```python
from build123d import *

# Parameters (mm, degrees)
BOSS_EXTRUDE1_DEPTH = 12.4
SKETCH2_R           = 1.5
CUT_EXTRUDE1_DEPTH  = 46.584756224
CUT_EXTRUDE2_DEPTH  = 2
CUT_EXTRUDE3_START  = -2
CUT_EXTRUDE3_DEPTH  = 2
CUT_EXTRUDE4_DEPTH  = 1
CUT_EXTRUDE5_START  = -1
CUT_EXTRUDE5_DEPTH  = 1
CUT_EXTRUDE6_DEPTH  = 0.5
SKETCH9_R           = 4.5
BOSS_EXTRUDE2_DEPTH = 0.5
SKETCH10_R          = 4.25
BOSS_EXTRUDE3_DEPTH = 0.5
SKETCH11_R          = 4.5
BOSS_EXTRUDE4_DEPTH = 1
SKETCH12_R          = 3
BOSS_EXTRUDE5_DEPTH = 1
SKETCH13_R          = 2
BOSS_EXTRUDE6_DEPTH = 3
BOSS_EXTRUDE7_DEPTH = 5


with BuildPart() as part:
    # Sketch1 → Boss-Extrude1 (new body)
    with BuildSketch(Plane(origin=(0, 0, 0), x_dir=(0, 0, -1), z_dir=(1, 0, 0))):
        with BuildLine():
            Line((1, 0), (27.9, 0))
            ThreePointArc((27.9, 0), (28.607106781, -0.292893219), (28.9, -1))
            Line((28.9, -1), (28.9, -24.904637595))
            ThreePointArc((28.9, -24.904637595), (28.813500063, -25.31147618), (28.568964732, -25.647931742))
            Line((28.568964732, -25.647931742), (20.685228726, -32.743294146))
            ThreePointArc((20.685228726, -32.743294146), (20.374527762, -32.933620412), (20.016263995, -33))
            Line((20.016263995, -33), (1, -33))
            ThreePointArc((1, -33), (0.292893219, -32.707106781), (0, -32))
            Line((0, -32), (0, -1))
            ThreePointArc((0, -1), (0.292893219, -0.292893219), (1, 0))
        make_face()
    extrude(amount=BOSS_EXTRUDE1_DEPTH)

    # Sketch2 → Cut-Extrude1 (cut, through all)
    with BuildSketch(Plane(origin=(12.4, 0, 0), x_dir=(0, 0, -1), z_dir=(1, 0, 0))):
        with Locations((25.9, -3)):
            Circle(SKETCH2_R)
        with Locations((9.9, -30)):
            Circle(SKETCH2_R)
    extrude(amount=-CUT_EXTRUDE1_DEPTH, mode=Mode.SUBTRACT)

    # Sketch3 → Cut-Extrude2 (cut)
    with BuildSketch(Plane(origin=(12.4, 0, 0), x_dir=(0, 0, -1), z_dir=(1, 0, 0))):
        with BuildLine():
            Line((6.9, -30), (6.9, -32.602246067))
            Line((6.9, -32.602246067), (0, -32.602246067))
            Line((0, -32.602246067), (0, -33))
            Line((0, -33), (6.9, -33))
            Line((6.9, -33), (12.9, -33))
            Line((12.9, -33), (12.9, -30))
            ThreePointArc((12.9, -30), (9.9, -27), (6.9, -30))
        make_face()
        with BuildLine():
            Line((22.9, 0), (28.9, 0))
            Line((28.9, 0), (28.9, -6))
            Line((28.9, -6), (25.9, -6))
            ThreePointArc((25.9, -6), (23.778679656, -5.121320344), (22.9, -3))
            Line((22.9, -3), (22.9, 0))
        make_face()
    extrude(amount=-CUT_EXTRUDE2_DEPTH, mode=Mode.SUBTRACT)

    # Sketch4 → Cut-Extrude3 (cut)
    with BuildSketch(Plane.ZY.offset(CUT_EXTRUDE3_START)):
        with BuildLine():
            Line((-12.9, -30), (-12.9, -33))
            Line((-12.9, -33), (-6.9, -33))
            Line((-6.9, -33), (0, -33))
            Line((0, -33), (0, -32.6))
            Line((0, -32.6), (-6.9, -32.6))
            Line((-6.9, -32.6), (-6.9, -30))
            ThreePointArc((-6.9, -30), (-9.9, -27), (-12.9, -30))
        make_face()
        with BuildLine():
            Line((-28.9, 0), (-22.9, 0))
            Line((-22.9, 0), (-22.9, -3))
            ThreePointArc((-22.9, -3), (-23.778679656, -5.121320344), (-25.9, -6))
            Line((-25.9, -6), (-28.9, -6))
            Line((-28.9, -6), (-28.9, 0))
        make_face()
    extrude(amount=CUT_EXTRUDE3_DEPTH, mode=Mode.SUBTRACT)

    # Sketch5 → Cut-Extrude4 (cut)
    with BuildSketch(Plane(origin=(12.4, 0, 0), x_dir=(0, 0, -1), z_dir=(1, 0, 0))):
        with BuildLine():
            Line((5, -3), (5, -25))
            ThreePointArc((5, -25), (5.292893219, -25.707106781), (6, -26))
            Line((6, -26), (10.9, -26))
            ThreePointArc((10.9, -26), (13.021320344, -26.878679656), (13.9, -29))
            Line((13.9, -29), (13.9, -30))
            Line((13.9, -30), (15.875361746, -30))
            ThreePointArc((15.875361746, -30), (16.233625514, -29.933620412), (16.544326478, -29.743294146))
            Line((16.544326478, -29.743294146), (27.068964732, -20.271119718))
            ThreePointArc((27.068964732, -20.271119718), (27.313500063, -19.934664157), (27.4, -19.527825572))
            Line((27.4, -19.527825572), (27.4, -8))
            ThreePointArc((27.4, -8), (27.107106781, -7.292893219), (26.4, -7))
            Line((26.4, -7), (24.9, -7))
            ThreePointArc((24.9, -7), (22.778679656, -6.121320344), (21.9, -4))
            Line((21.9, -4), (21.9, -3))
            ThreePointArc((21.9, -3), (21.607106781, -2.292893219), (20.9, -2))
            Line((20.9, -2), (6, -2))
            ThreePointArc((6, -2), (5.292893219, -2.292893219), (5, -3))
        make_face()
    extrude(amount=-CUT_EXTRUDE4_DEPTH, mode=Mode.SUBTRACT)

    # Sketch6 → Cut-Extrude5 (cut)
    with BuildSketch(Plane.ZY.offset(CUT_EXTRUDE5_START)):
        with BuildLine():
            Line((-6, -2), (-20.9, -2))
            ThreePointArc((-20.9, -2), (-21.607106781, -2.292893219), (-21.9, -3))
            Line((-21.9, -3), (-21.9, -4))
            ThreePointArc((-21.9, -4), (-22.778679656, -6.121320344), (-24.9, -7))
            Line((-24.9, -7), (-26.4, -7))
            ThreePointArc((-26.4, -7), (-27.107106781, -7.292893219), (-27.4, -8))
            Line((-27.4, -8), (-27.4, -19.527825572))
            ThreePointArc((-27.4, -19.527825572), (-27.313500063, -19.934664157), (-27.068964732, -20.271119718))
            Line((-27.068964732, -20.271119718), (-16.544326478, -29.743294146))
            ThreePointArc((-16.544326478, -29.743294146), (-16.233625514, -29.933620412), (-15.875361746, -30))
            Line((-15.875361746, -30), (-13.9, -30))
            Line((-13.9, -30), (-13.9, -29))
            ThreePointArc((-13.9, -29), (-13.021320344, -26.878679656), (-10.9, -26))
            Line((-10.9, -26), (-6, -26))
            ThreePointArc((-6, -26), (-5.292893219, -25.707106781), (-5, -25))
            Line((-5, -25), (-5, -3))
            ThreePointArc((-5, -3), (-5.292893219, -2.292893219), (-6, -2))
        make_face()
    extrude(amount=CUT_EXTRUDE5_DEPTH, mode=Mode.SUBTRACT)

    # Sketch8 → Cut-Extrude6 (cut)
    with BuildSketch(Plane.XY):
        with BuildLine():
            Line((3.6, -3.5), (9.6, -3.5))
            ThreePointArc((9.6, -3.5), (10.307106781, -3.792893219), (10.6, -4.5))
            Line((10.6, -4.5), (10.6, -13.5))
            ThreePointArc((10.6, -13.5), (10.307106781, -14.207106781), (9.6, -14.5))
            Line((9.6, -14.5), (3.6, -14.5))
            ThreePointArc((3.6, -14.5), (2.892893219, -14.207106781), (2.6, -13.5))
            Line((2.6, -13.5), (2.6, -4.5))
            ThreePointArc((2.6, -4.5), (2.892893219, -3.792893219), (3.6, -3.5))
        make_face()
        with BuildLine():
            Line((3.6, -17.7), (9.6, -17.7))
            ThreePointArc((9.6, -17.7), (10.307106781, -17.992893219), (10.6, -18.7))
            Line((10.6, -18.7), (10.6, -29))
            ThreePointArc((10.6, -29), (10.307106781, -29.707106781), (9.6, -30))
            Line((9.6, -30), (3.6, -30))
            ThreePointArc((3.6, -30), (2.892893219, -29.707106781), (2.6, -29))
            Line((2.6, -29), (2.6, -18.7))
            ThreePointArc((2.6, -18.7), (2.892893219, -17.992893219), (3.6, -17.7))
        make_face()
    extrude(amount=-CUT_EXTRUDE6_DEPTH, mode=Mode.SUBTRACT)

    # Sketch9 → Boss-Extrude2 (add)
    with BuildSketch(Plane(origin=(0, 0, -28.9), x_dir=(-1, 0, 0), z_dir=(0, 0, -1))):
        with Locations(Location((-6.9, -15, 0), (0, 0, 270))):
            Circle(SKETCH9_R)
    extrude(amount=BOSS_EXTRUDE2_DEPTH)

    # Sketch10 → Boss-Extrude3 (add)
    with BuildSketch(Plane(origin=(0, 0, -29.4), x_dir=(-1, 0, 0), z_dir=(0, 0, -1))):
        with Locations(Location((-6.9, -15, 0), (0, 0, 90))):
            Circle(SKETCH10_R)
    extrude(amount=BOSS_EXTRUDE3_DEPTH)

    # Sketch11 → Boss-Extrude4 (add)
    with BuildSketch(Plane(origin=(0, 0, -29.9), x_dir=(-1, 0, 0), z_dir=(0, 0, -1))):
        with Locations(Location((-6.9, -15, 0), (0, 0, 270))):
            Circle(SKETCH11_R)
    extrude(amount=BOSS_EXTRUDE4_DEPTH)

    # Sketch12 → Boss-Extrude5 (add)
    with BuildSketch(Plane(origin=(0, -28.375690608, -25.538121547), x_dir=(1, 0, 0), z_dir=(0, -0.7432941462471664, -0.6689647316224496))):
        with Locations(Location((6.2, 1.22565854, 0), (0, 0, 90))):
            Circle(SKETCH12_R)
    extrude(amount=BOSS_EXTRUDE5_DEPTH)

    # Sketch13 → Boss-Extrude6 (add)
    with BuildSketch(Plane(origin=(0, -29.118984754, -26.207086279), x_dir=(1, 0, 0), z_dir=(0, -0.7432941462471664, -0.6689647316224496))):
        with Locations(Location((6.2, 1.22565854, 0), (0, 0, 270))):
            Circle(SKETCH13_R)
    extrude(amount=BOSS_EXTRUDE6_DEPTH)

    # Sketch14 → Boss-Extrude7 (add)
    with BuildSketch(Plane(origin=(0, -31.348867193, -28.213980473), x_dir=(1, 0, 0), z_dir=(0, -0.7432941462471664, -0.6689647316224496))):
        with BuildLine():
            ThreePointArc((6.21, 1.126159796), (7.2, 1.22565854), (6.21, 1.325157284))
            ThreePointArc((6.21, 1.325157284), (5.22, 1.22565854), (6.21, 1.126159796))
        make_face()
    extrude(amount=BOSS_EXTRUDE7_DEPTH)


solid = part.part
```
Design review of the part built by this model. Coordinates are the model's own, in mm. A direction names the side the tool comes from. Give positions to 0.01 mm unless a question says otherwise; leave off trailing zeros. Loops run counter-clockwise (first coordinate to the right, second up) from the corner with the lowest first, then second, coordinate; pieces in that order, holes last. Notation, with made-up numbers: (-38.75, 2.5) -> (-22.75, 2.5) arc R19 cw to (-22.75, 18.5) -> close; hole circle Ø6 at (-34, 19). An arc over 180 degrees is marked (long way). Write each question's results on one line, items separated by ' | '.
Q1. Take a section at A-A, the plane z = -9.9. Write out the cut boundary in (x, y), plus the area to 3 significant figures.
Reply:
outline: (0, -27) -> (2, -27) -> (2, -28.5) -> (10.4, -28.5) -> (10.4, -27) -> (12.4, -27) -> (12.4, -26) -> (11.4, -26) -> (11.4, -2) -> (12.4, -2) -> (12.4, 0) -> (0, 0) -> (0, -2) -> (1, -2) -> (1, -26) -> (0, -26) -> close; (2, -33) -> (10.4, -33) -> (10.4, -31.5) -> (2, -31.5) -> close | area: 312 mm²
Q2. The part is to be moulded in two halves that separate along Z. For faces 1 (the face through (11.41, -5.14, -23.8)), 2 (the face through (0.507, -2.301, -5.285)), 3 (the face through (10.315, -29.699, -0.246)), say which applies: +Z half, -Z half, draft (parallel to the pull), parting line (faces both ways), or undercut.
Reply:
face 1: -Z half | face 2: undercut | face 3: draft
Q3. For pin 1 Ø2.5 at (x, y) = (8, -7) entering from +Z; pin 2 Ø1.5 at (y, z) = (-19, -7) entering from -X; pin 3 Ø4 at (x, y) = (5.5, -10.5) entering from -Z; pin 4 Ø2.5 at (y, z) = (-30, -9.9) entering from -X, all flat-tipped, find the tip position at first contact; note any pin that passes through.
Reply:
pin 1: stops at z = -0.5 | pin 2: stops at x = 1 | pin 3: stops at z = -30.9 | pin 4: passes through
Q4. Take a section at D-D, the plane x = 5.75. Give the number of separate pieces and of enclosed holes in the cut face, plus the area to 3 significant figures.
Reply:
separate pieces: 1 | enclosed holes: 2 | area: 934 mm²
Q5. Take a section at B-B, the plane y = -15. Write out the cut boundary in (x, z).
Reply:
outline: (0, -28.9) -> (2.4, -28.9) -> (2.4, -29.4) -> (2.65, -29.4) -> (2.65, -29.9) -> (2.4, -29.9) -> (2.4, -30.9) -> (11.4, -30.9) -> (11.4, -29.9) -> (11.15, -29.9) -> (11.15, -29.4) -> (11.4, -29.4) -> (11.4, -28.9) -> (12.4, -28.9) -> (12.4, -27.4) -> (11.4, -27.4) -> (11.4, -5) -> (12.4, -5) -> (12.4, 0) -> (0, 0) -> (0, -5) -> (1, -5) -> (1, -27.4) -> (0, -27.4) -> close
Q6. Machinability: for faces 4 (the face through (1, -1, -22.9)), 5 (the face through (1, -31, -12.9)), 6 (the face through (0.51, -26.9, -13.04)), which of the approach directions +Z, -Z, +X, -X, +Y, -Y give a long, thin tool a straight path to every point of the face, cutting with its end or side? Answer none if there is none.
Reply:
face 4: -Z, -X, +Y | face 5: -X, -Y | face 6: -X
Q7. Take a section at C-C, the plane z = -3. Write out the cut boundary in (x, y), plus the area to 3 significant figures.
Reply:
outline: (0, -32.6) -> (2, -32.6) -> (2, -33) -> (10.4, -33) -> (10.4, -32.6) -> (12.4, -32.6) -> (12.4, 0) -> (0, 0) -> close | area: 408 mm²
Q8. Wall thickness on L1, parallel to Y at x = 5.75, z = -9.9; L2, parallel to X at y = -24, z = -8.5; L3, parallel to Y at x = 4, z = -16: over which ranges is each line inside the solid? List them lowest first.
Reply:
L1: y = -33 to -31.5, -28.5 to 0 | L2: x = 1 to 11.4 | L3: y = -33 to 0
